```python
from build123d import *

# Parameters (mm, degrees)
SKETCH1_W             = 249
SKETCH1_H             = 195
SKETCH1_R             = 1.95
BOSS_EXTRUDE1_DEPTH   = 19.05
M6X1_0_TAPPED_HOLE1_D = 5
F_8_0MM_DOWEL_HOLE1_D = 8


with BuildPart() as part:
    # Sketch1 → Boss-Extrude1 (new body)
    with BuildSketch(Plane(origin=(0, 0, 0), x_dir=(1, 0, 0), z_dir=(0, 1, 0))):
        with Locations((54.5, 53.449182879)):
            Rectangle(SKETCH1_W, SKETCH1_H)
        with Locations(Location((-30, -9.050817121, 0), (0, 0, 90))):
            Circle(SKETCH1_R, mode=Mode.SUBTRACT)
        with Locations(Location((0, -9.050817121, 0), (0, 0, 90))):
            Circle(SKETCH1_R, mode=Mode.SUBTRACT)
        with Locations(Location((0, -34.050817121, 0), (0, 0, 90))):
            Circle(SKETCH1_R, mode=Mode.SUBTRACT)
        with Locations(Location((-30, -34.050817121, 0), (0, 0, 90))):
            Circle(SKETCH1_R, mode=Mode.SUBTRACT)
        with Locations(Location((109, -34.050817121, 0), (0, 0, 90))):
            Circle(SKETCH1_R, mode=Mode.SUBTRACT)
        with Locations(Location((109, -9.050817121, 0), (0, 0, 90))):
            Circle(SKETCH1_R, mode=Mode.SUBTRACT)
        with Locations(Location((139, -9.050817121, 0), (0, 0, 90))):
            Circle(SKETCH1_R, mode=Mode.SUBTRACT)
        with Locations(Location((139, -34.050817121, 0), (0, 0, 90))):
            Circle(SKETCH1_R, mode=Mode.SUBTRACT)
        with Locations(Location((109, 115.949182879, 0), (0, 0, 90))):
            Circle(SKETCH1_R, mode=Mode.SUBTRACT)
        with Locations(Location((109, 140.949182879, 0), (0, 0, 90))):
            Circle(SKETCH1_R, mode=Mode.SUBTRACT)
        with Locations(Location((139, 140.949182879, 0), (0, 0, 90))):
            Circle(SKETCH1_R, mode=Mode.SUBTRACT)
        with Locations(Location((139, 115.949182879, 0), (0, 0, 90))):
            Circle(SKETCH1_R, mode=Mode.SUBTRACT)
        with Locations(Location((-30, 115.949182879, 0), (0, 0, 90))):
            Circle(SKETCH1_R, mode=Mode.SUBTRACT)
        with Locations(Location((-30, 140.949182879, 0), (0, 0, 90))):
            Circle(SKETCH1_R, mode=Mode.SUBTRACT)
        with Locations(Location((0, 140.949182879, 0), (0, 0, 90))):
            Circle(SKETCH1_R, mode=Mode.SUBTRACT)
        with Locations(Location((0, 115.949182879, 0), (0, 0, 90))):
            Circle(SKETCH1_R, mode=Mode.SUBTRACT)
    extrude(amount=BOSS_EXTRUDE1_DEPTH)

    # M6x1.0 Tapped Hole1 (through all)
    with Locations(Plane(origin=(0, 19.05, 0), x_dir=(1, 0, 0), z_dir=(0, 1, 0))):
        with Locations((-36.092306809, 37.249182879), (143.907693191, 37.249182879), (143.907693191, -22.750817121), (-36.092306809, -22.750817121)):
            Hole(M6X1_0_TAPPED_HOLE1_D / 2)

    # Ø8.0mm Dowel Hole1 (through all)
    with Locations(Plane(origin=(0, 19.05, 0), x_dir=(1, 0, 0), z_dir=(0, 1, 0))):
        with Locations((53.907693191, 7.249182879)):
            Hole(F_8_0MM_DOWEL_HOLE1_D / 2)


solid = part.part
```
The model under review builds one solid part; all positions refer to its coordinate system, in mm. Round coordinates to 2 decimals unless told otherwise and drop trailing zeros. Answer as a JSON object with one key per item and string values. Group by question number.
1) Mouldability with a two-part tool opening along X and no side actions: class faces 1 (the face through (-37.436, 9.392, -39.357)), 2 (the face through (53, 9, -150.949)), 3 (the face through (-70, 9, -52)) as released by +X, released by -X, zero draft, split by the parting line, or undercut.
2) For line 1 (Z direction, x = 139, y = 5.25); line 2 (Z direction, x = 56, y = 10.25), list the stretches that pass through material, from the lowest coordinate up. Write a range as [from, to].
3) For pin 1 Ø3.5 at (x, z) = (139, 9.05) entering from -Y, flat-tipped, find the tip position at first contact; note if it passes through.
Result set:
{
 "1": {"face 1": "undercut", "face 2": "zero draft", "face 3": "released by -X"},
 "2": {"line 1": "[-150.95, -142.9], [-139, -117.9], [-114, 7.1], [11, 32.1], [36, 44.05]", "line 2": "[-150.95, -10.66], [-3.84, 44.05]"},
 "3": {"pin 1": "through"}
}
